Verification items for the finished model (mm, model axes). Face numbers are marked on the shaded views. A direction names the side the tool comes from. Give positions to 0.01 mm unless a question says otherwise; leave off trailing zeros. Loops run counter-clockwise (first coordinate to the right, second up) from the corner with the lowest first, then second, coordinate; pieces in that order, holes last. Notation, with made-up numbers: (76.25, 15) - (118.25, 15) arc R17 cw to (118.25, 26) - close; hole circle Ø2 at (-30.5, -39.75). An arc over 180 degrees is marked (long way). Answer in a Markdown table with one row per item.
```python
from build123d import *

# Parameters (mm, degrees)
BOSS_EXTRUDE3_DEPTH = 1.8
SKETCH3_R           = 2.45
BOSS_EXTRUDE4_DEPTH = 0.6
SKETCH4_R           = 2.2
CUT_EXTRUDE1_DEPTH  = 1.3
SKETCH5_R           = 0.8
CUT_EXTRUDE2_DEPTH  = 3
BOSS_EXTRUDE5_START = 2.2
SKETCH6_R           = 3
BOSS_EXTRUDE5_DEPTH = 2.2
SKETCH7_R           = 1.9
CUT_EXTRUDE3_DEPTH  = 2.5


with BuildPart() as part:
    # Sketch1 → Boss-Extrude3 (new body)
    with BuildSketch(Plane(origin=(0, 0, 0), x_dir=(1, 0, 0), z_dir=(0, 1, 0))):
        with BuildLine():
            Line((-3, 0), (-1.95, 13))
            ThreePointArc((-1.95, 13), (0, 14.95), (1.95, 13))
            Line((1.95, 13), (3, 0))
            ThreePointArc((3, 0), (0, -3), (-3, 0))
        make_face()
    extrude(amount=BOSS_EXTRUDE3_DEPTH)

    # Sketch3 → Boss-Extrude4 (add)
    with BuildSketch(Plane(origin=(0, 1.8, 0), x_dir=(1, 0, 0), z_dir=(0, 1, 0))):
        with Locations(Location((0, 0, 0), (0, 0, 270))):
            Circle(SKETCH3_R)
    extrude(amount=BOSS_EXTRUDE4_DEPTH)

    # Sketch4 → Cut-Extrude1 (cut)
    with BuildSketch(Plane(origin=(0, 2.4, 0), x_dir=(1, 0, 0), z_dir=(0, 1, 0))):
        with Locations(Location((0, 0, 0), (0, 0, 270))):
            Circle(SKETCH4_R)
    extrude(amount=-CUT_EXTRUDE1_DEPTH, mode=Mode.SUBTRACT)

    # Sketch5 → Cut-Extrude2 (cut)
    with BuildSketch(Plane(origin=(0, 1.1, 0), x_dir=(1, 0, 0), z_dir=(0, 1, 0))):
        with Locations(Location((0, 0, 0), (0, 0, 270))):
            Circle(SKETCH5_R)
    extrude(amount=-CUT_EXTRUDE2_DEPTH, mode=Mode.SUBTRACT)

    # Sketch6 → Boss-Extrude5 (add)
    with BuildSketch(Plane.XZ.offset(BOSS_EXTRUDE5_START)):
        with Locations(Location((0, 0, 0), (0, 0, 270))):
            Circle(SKETCH6_R)
    extrude(amount=-BOSS_EXTRUDE5_DEPTH)

    # Sketch7 → Cut-Extrude3 (cut)
    with BuildSketch(Plane.XZ.offset(2.2)):
        with Locations(Location((0, 0, 0), (0, 0, 270))):
            Circle(SKETCH7_R)
    extrude(amount=-CUT_EXTRUDE3_DEPTH, mode=Mode.SUBTRACT)


solid = part.part
```
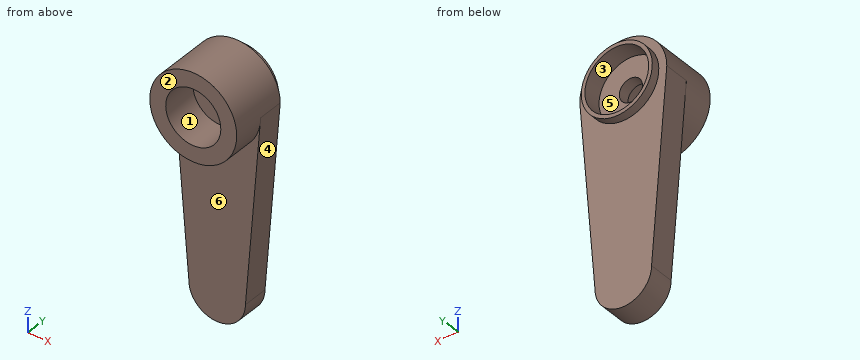
Q1. Sectioned sample at D-D (x = 1.25). Record the cut outline in (y, z), and give its area (3 significant figures).
Completed:
| item | result |
|---|---|
| outline | (-2.2, -2.73) - (0, -2.73) - (0, -14.5) - (1.8, -14.5) - (1.8, -2.11) - (2.4, -2.11) - (2.4, -1.81) - (1.1, -1.81) - (1.1, 1.81) - (2.4, 1.81) - (2.4, 2.11) - (1.8, 2.11) - (1.8, 2.73) - (-2.2, 2.73) - (-2.2, 1.43) - (0.3, 1.43) - (0.3, -1.43) - (-2.2, -1.43) - close |
| area | 33.7 mm^2 |
Q2. Thickness scan on line 1 (X direction, y = 1.9, z = 0); line 2 (Y direction, x = 0.45, z = 1.25); line 3 (Y direction, x = 0.95, z = -5.5). Record the ranges inside material, lowest first.
Completed:
| item | result |
|---|---|
| line 1 | -2.45 to -2.2, 2.2 to 2.45 |
| line 2 | 0.3 to 1.1 |
| line 3 | 0 to 1.8 |
Q3. Draft check along Z on the marked faces 4, 5 and 6. Enter one of: +Z half, -Z half, draft (parallel to the pull), parting line (faces both ways), or undercut.
Completed:
| item | result |
|---|---|
| face 4 | -Z half |
| face 5 | undercut |
| face 6 | draft |
Q4. Go/stop test with flat-tipped pins: P1, Ø1, axis at x = 0, z = -4.5, coming from the -Y side; P2, Ø2, axis at x = 0, z = 0, coming from the -Y side. Record where each tip stops, or that it passes through.
Completed:
| item | result |
|---|---|
| P1 | y = 0 |
| P2 | y = 0.3 |
Q5. Sectioned sample at A-A (x = 0). Record the cut outline in (y, z).
Completed:
| item | result |
|---|---|
| outline | (-2.2, -3) - (0, -3) - (0, -14.95) - (1.8, -14.95) - (1.8, -2.45) - (2.4, -2.45) - (2.4, -2.2) - (1.1, -2.2) - (1.1, -0.8) - (0.3, -0.8) - (0.3, -1.9) - (-2.2, -1.9) - close; (-2.2, 1.9) - (0.3, 1.9) - (0.3, 0.8) - (1.1, 0.8) - (1.1, 2.2) - (2.4, 2.2) - (2.4, 2.45) - (1.8, 2.45) - (1.8, 3) - (-2.2, 3) - close |
Q6. Sectioned sample at B-B (y = -1.4). Record the cut outline in (x, z).
Completed:
| item | result |
|---|---|
| outline | circle Ø6 at (0, 0); hole circle Ø3.8 at (0, 0) |
Q7. Sectioned sample at C-C (z = 1). Record the cut outline in (x, y), and give its area (3 significant figures).
Completed:
| item | result |
|---|---|
| outline | (-2.83, -2.2) - (-1.62, -2.2) - (-1.62, 0.3) - (1.62, 0.3) - (1.62, -2.2) - (2.83, -2.2) - (2.83, 1.8) - (2.24, 1.8) - (2.24, 2.4) - (1.96, 2.4) - (1.96, 1.1) - (-1.96, 1.1) - (-1.96, 2.4) - (-2.24, 2.4) - (-2.24, 1.8) - (-2.83, 1.8) - close |
| area | 12.1 mm^2 |
Q8. Tool access check on the marked faces 1, 2 and 3. Record the directions out of +Z, -Z, +X, -X, +Y, -Y that give a thin tool (end or side, any length) a straight path to the whole face; none if there is none.
Completed:
| item | result |
|---|---|
| face 1 | -Y |
| face 2 | +Z, -Z, +X, -X, -Y |
| face 3 | +Y |
